For this review, take the finished solid that the model builds, in its own axes (mm). A direction names the side the tool comes from. Round coordinates to 2 decimals unless told otherwise and drop trailing zeros. Write each loop counter-clockwise with the first axis right and the second up, starting at its lowest first coordinate (ties: lowest second). Pieces come first, ordered by that corner, then holes. Notation, with made-up numbers: (82.5, 82) - (93.5, 82) arc R28 ccw to (93.5, 118) - close; hole circle Ø3 at (23, 18.25). An arc over 180 degrees is marked (long way). One line per item, written item: value. Start each with the question number.
Q1. Clearance check with flat-ended pins moving along their axes: pin 1 Ø2 at (x, z) = (-101.5, 9) entering from -Y; pin 2 Ø3.5 at (x, y) = (-72, 185) entering from -Z; pin 3 Ø1.8 at (x, y) = (-37.5, 160.55) entering from -Z; pin 4 Ø8 at (x, z) = (-59.5, 12) entering from +Y. State where each tip first meets the part, or that it passes through.
Q2. Add section D-D on y = 181.75. Write out the cut boundary in (x, z).
Q3. Add section B-B on y = 160.55. Write out the cut boundary in (x, z), and give its area (3 significant figures).
Q4. Add section C-C on x = -92. Write out the cut boundary in (y, z).
Q5. Mouldability with a two-part tool opening along Z and no side actions: class faces 4 (the face through (-73, 164, 18.45)), 5 (the face through (-74, 173, 7)), 6 (the face through (-78, 158.05, 19)) as +Z half, -Z half, draft (parallel to the pull), parting line (faces both ways), or undercut.
Q6. Add section A-A on x = -37.5. Write out the cut boundary in (y, z).
Q7. Tool access review of faces 1 (the face through (-73, 165.8, 11)), 2 (the face through (-73, 183, 18.45)), 3 (the face through (-73, 167, 14.15)): name each direction out of +Z, -Z, +X, -X, +Y, -Y from which nothing blocks a thin tool from reaching the whole face with its end or side.
Q8. For probe 1 along X at (y, z) = (185.55, 19.4); probe 2 along Y at (x, z) = (-37.5, 20.8); probe 3 along Y at (x, z) = (-42.5, 17.75), list the stretches that pass through material, from the lowest coordinate up.
```python
from build123d import *

# Parameters (mm, degrees)
PAD113_DEPTH    = 85
SKETCH229_R     = 1.5
POCKET082_DEPTH = 15.451
SKETCH230_W     = 30
SKETCH230_H     = 15.45
PAD114_DEPTH    = 4


with BuildPart() as part:
    # Sketch228 → Pad113 (new body)
    with BuildSketch(Plane.YZ):
        Polygon((-7.75, 11.45), (-7.75, 15.45), (22.25, 15.45), (22.25, 11.45), (11.25, 11.45), (11.25, 7.15), (14.5, 7.15), (14.5, 0), (0, 0), (0, 7.15), (3.25, 7.15), (3.25, 11.45), align=None)
    extrude(amount=PAD113_DEPTH)

    # Sketch229 (on Face2 of Pad113) → Pocket082 (cut, through all)
    with BuildSketch(Plane(origin=(0, 0, 15.45), x_dir=(0, -1, 0), z_dir=(0, 0, 1))):
        with Locations((-19.75, 77.5)):
            Circle(SKETCH229_R)
        with Locations((-19.75, 52.5)):
            Circle(SKETCH229_R)
        with Locations((5.25, 52.5)):
            Circle(SKETCH229_R)
        with Locations((5.25, 77.5)):
            Circle(SKETCH229_R)
    extrude(amount=-POCKET082_DEPTH, mode=Mode.SUBTRACT)

    # Sketch230 (on Face4 of Pocket082) → Pad114 (join)
    with BuildSketch(Plane(origin=(0, 0, 0), x_dir=(0, 1, 0), z_dir=(-1, 0, 0))):
        with Locations((7.25, -7.725)):
            Rectangle(SKETCH230_W, SKETCH230_H)
    extrude(amount=PAD114_DEPTH)


with BuildPart() as part_1:
    # Body136 placement: moved
    add(part.part.moved(Location((-115, 165.8, 7))))


solid = part_1.part
```
Result set:
1. pin 1: stops at y = 165.8
1. pin 2: stops at z = 18.45
1. pin 3: passes through
1. pin 4: stops at y = 180.3
2. outline: (-119, 7) - (-115, 7) - (-115, 18.45) - (-30, 18.45) - (-30, 22.45) - (-119, 22.45) - close
3. outline: (-119, 7) - (-115, 7) - (-115, 18.45) - (-64, 18.45) - (-64, 22.45) - (-119, 22.45) - close; (-61, 18.45) - (-39, 18.45) - (-39, 22.45) - (-61, 22.45) - close; (-36, 18.45) - (-30, 18.45) - (-30, 22.45) - (-36, 22.45) - close
3. area: 378 mm^2
4. outline: (158.05, 18.45) - (169.05, 18.45) - (169.05, 14.15) - (165.8, 14.15) - (165.8, 7) - (180.3, 7) - (180.3, 14.15) - (177.05, 14.15) - (177.05, 18.45) - (188.05, 18.45) - (188.05, 22.45) - (158.05, 22.45) - close
5. face 4: undercut
5. face 5: -Z half
5. face 6: draft
6. outline: (158.05, 18.45) - (159.05, 18.45) - (159.05, 22.45) - (158.05, 22.45) - close; (162.05, 18.45) - (169.05, 18.45) - (169.05, 14.15) - (165.8, 14.15) - (165.8, 7) - (180.3, 7) - (180.3, 14.15) - (177.05, 14.15) - (177.05, 18.45) - (184.05, 18.45) - (184.05, 22.45) - (162.05, 22.45) - close; (187.05, 18.45) - (188.05, 18.45) - (188.05, 22.45) - (187.05, 22.45) - close
7. face 1: -Z, +X, -Y
7. face 2: +X, +Y
7. face 3: +X, -Y
8. probe 1: x = -119 to -64, -61 to -39, -36 to -30
8. probe 2: y = 158.05 to 159.05, 162.05 to 184.05, 187.05 to 188.05
8. probe 3: y = 169.05 to 177.05
